CAD build for the part. Positions are in the model's coordinates, mm. A direction names the side the tool comes from. Give positions to 0.01 mm unless a question says otherwise; leave off trailing zeros. Write each loop counter-clockwise with the first axis right and the second up, starting at its lowest first coordinate (ties: lowest second). Pieces come first, ordered by that corner, then holes. Notation, with made-up numbers: (12, -32) -> (22, -32) arc R17 cw to (22, -9) -> close; hole circle Ø5 at (-3.5, 15). An arc over 180 degrees is marked (long way). Answer as a JSON object with one key per item and string values.
```python
from build123d import *

# Parameters (mm, degrees)
F0_W     = 21.59
F0_H     = 25.4
F1_DEPTH = 25.4
F2_DEPTH = 27.94
F3_DEPTH = 25.4


with BuildPart() as f1:
    # F0 (on Top) → F1 (new body)
    with BuildSketch(Plane.XY):
        with Locations((-10.795, 51.474535)):
            Rectangle(F0_W, F0_H)
        Polygon((-24.402696, 34.54427), (6.066474, 34.54427), (0, 38.774535), (-21.59, 38.774535), align=None)
    extrude(amount=F1_DEPTH)

    # F0 (on Top) → F2 (join)
    with BuildSketch(Plane.XY):
        Polygon((-10.795, 0), (0, 0), (6.066474, 0), (6.066474, 34.54427), (-24.402696, 34.54427), (-24.402696, 0), (-21.59, 0), align=None)
    extrude(amount=F2_DEPTH)

    # F0 (on Top) → F3 (join)
    with BuildSketch(Plane.XY):
        Polygon((6.066474, 0), (0, 0), (-10.795, 0), (-21.59, 0), (-24.402696, 0), (-24.402696, -17.78), (-17.076401, -55.168974), (-10.795, -67.434295), (-1.259822, -55.168974), (6.066474, -17.78), align=None)
    extrude(amount=F3_DEPTH)


solid = f1.part
```
1) Pin check, flat tips, straight feed: pin 1 (0.8 mm diameter, centred on x = -14.5, z = 27, fed in from -Y); pin 2 (2 mm diameter, centred on x = 2, y = -6, fed in from +Z); pin 3 (10 mm diameter, centred on x = -2, y = 47.5, fed in from -Z); pin 4 (3 mm diameter, centred on y = -24.5, z = 11.5, fed in from +X). Stop position of each tip, or through.
Model answer:
{"pin 1": "stops at y = 0", "pin 2": "stops at z = 25.4", "pin 3": "stops at z = 0", "pin 4": "stops at x = 5.04"}
2) 3-axis set-ups, long thin cutter, end or side, ignore diameter. For faces 1 (the flat face through (-21.59, 51, 13)), 2 (the flat face through (-9, -26, 25.4)), 3 (the flat face through (0, 51, 13)): which of +Z, -Z, +X, -X, +Y, -Y reach the whole face in a straight line?
Model answer:
{"face 1": "+Z, -Z, -X, +Y", "face 2": "+Z, +X, -X, -Y", "face 3": "+Z, -Z, +X, +Y"}
3) Slice it at C-C (y = -13). List the corners of the cut face in (x, z).
Model answer:
{"outline": "(-24.4, 0) -> (6.07, 0) -> (6.07, 25.4) -> (-24.4, 25.4) -> close"}
4) Slice it at A-A (z = 21.75). List the corners of the cut face in (x, y) (3 decimals).
Model answer:
{"outline": "(-24.403, -17.78) -> (-17.076, -55.169) -> (-10.795, -67.434) -> (-1.26, -55.169) -> (6.066, -17.78) -> (6.066, 34.544) -> (0, 38.775) -> (0, 64.175) -> (-21.59, 64.175) -> (-21.59, 38.775) -> (-24.403, 34.544) -> close"}
5) Slice it at B-B (x = 3). List the corners of the cut face in (y, z).
Model answer:
{"outline": "(-33.43, 0) -> (36.68, 0) -> (36.68, 25.4) -> (34.54, 25.4) -> (34.54, 27.94) -> (0, 27.94) -> (0, 25.4) -> (-33.43, 25.4) -> close"}
6) Slice it at D-D (y = -53). List the corners of the cut face in (x, z), then the cut area to 3 significant figures.
Model answer:
{"outline": "(-17.5, 0) -> (-0.83, 0) -> (-0.83, 25.4) -> (-17.5, 25.4) -> close", "area": "423 mm2"}
7) Wall check: probe 1 along Z at (x, y) = (-21, 41); probe 2 along X at (y, z) = (56, 16); probe 3 along Y at (x, z) = (-4.5, 25). Give the ranges that are in metal, low to high.
Model answer:
{"probe 1": "z = 0 to 25.4", "probe 2": "x = -21.59 to 0", "probe 3": "y = -59.34 to 64.17"}
